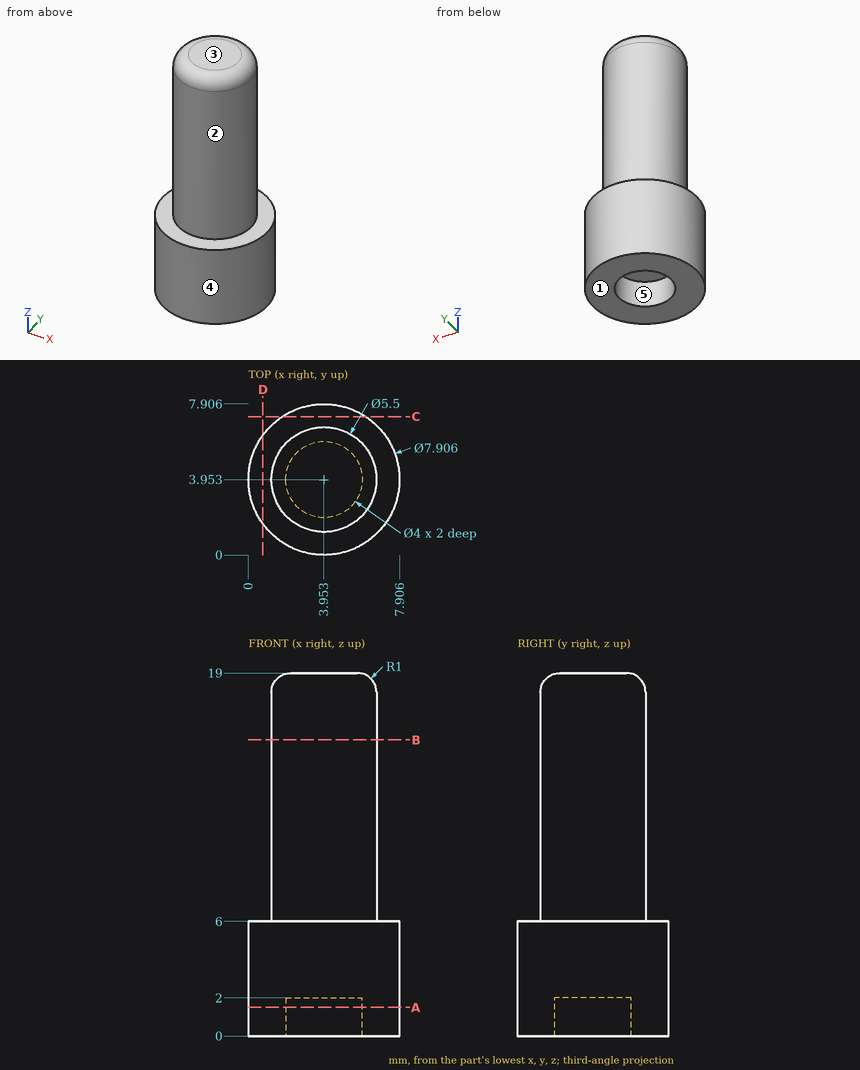
Geometry check sheet. Reference: drawing and pictorial views, mm from the part's lowest x, y, z. A direction names the side the tool comes from. Round coordinates to 2 decimals unless told otherwise and drop trailing zeros. Loops run counter-clockwise (first coordinate to the right, second up) from the corner with the lowest first, then second, coordinate; pieces in that order, holes last. Notation, with made-up numbers: M 28.5,-39.5 L 57.5,-39.5 A27 ccw 57.5,-15.5 Z; hole C 44,-7 d2. An arc over 180 degrees is marked long. One line per item, written item: value.
(1) Thickness scan on line 1 (Z direction, x = 7, y = 2); line 2 (Z direction, x = 4.5, y = 2.5); line 3 (Y direction, x = 2.5, z = 1.5) (1 decimal). Record the ranges inside material, lowest first.
Computed values:
line 1: z = 0 to 6
line 2: z = 2 to 19
line 3: y = 0.3 to 2.6, 5.3 to 7.6
(2) Release check for a two-part mould opening along Y. For the marked faces 3, 4 and 5 record: +Y half, -Y half, draft (parallel to the pull), parting line (faces both ways), or undercut.
Computed values:
face 3: draft
face 4: parting line
face 5: undercut
(3) Sectioned sample at A-A, the plane z = 1.5. Record the cut outline in (x, y).
Computed values:
outline: C 3.95,3.95 d7.91; hole C 3.95,3.95 d4
(4) Access from +Z, -Z, +X, -X, +Y, -Y to the whole of each face (thin tool, end or side, straight path). Record for the marked faces 1 and 2.
Computed values:
face 1: -Z, +X, -X, +Y, -Y
face 2: +Z
(5) Sectioned sample at D-D, the plane x = 0.75. Record the cut outline in (y, z).
Computed values:
outline: M 1.64,0 L 6.27,0 L 6.27,6 L 1.64,6 Z
(6) Sectioned sample at C-C, the plane y = 7.25. Record the cut outline in (x, z).
Computed values:
outline: M 1.77,0 L 6.13,0 L 6.13,6 L 1.77,6 Z
(7) Sectioned sample at B-B, the plane z = 15.5. Record the cut outline in (x, y).
Computed values:
outline: C 3.95,3.95 d5.5
(8) Depth check by flat-ended pin: pin 1 Ø1.5 at (x, z) = (7, 7) entering from -Y; pin 2 Ø3 at (y, z) = (6.5, 2.5) entering from +X (1 decimal); pin 3 Ø1.5 at (x, z) = (4.5, 11.5) entering from +Y. Enter the tip coordinate at first touch or a pass-through.
Computed values:
pin 1: stops at y = 2.44
pin 2: stops at x = 7.8
pin 3: stops at y = 6.7
